Design review of the part built by this model. Coordinates are the model's own, in mm. Round coordinates to 2 decimals unless told otherwise and drop trailing zeros. Order: outer loops, then holes, each group sorted by start corner. A loop starts at its lowest first (then second) coordinate and runs counter-clockwise, first axis right, second up. Notation, with made-up numbers: (-24.5, 34.5) - (26.5, 34.5) arc R14 cw to (26.5, 55.5) - close; hole circle Ø5 at (41, 45.25). An arc over 180 degrees is marked (long way). Write item = value, one per line.
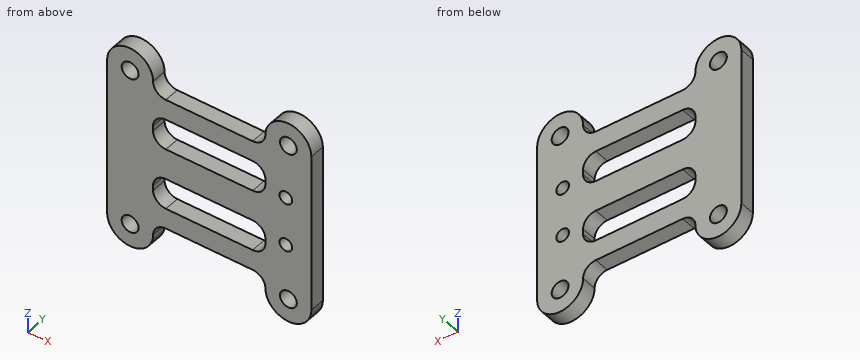
from build123d import *

# Parameters (mm, degrees)
F0_R     = 1.65
F0_R_2   = 1.25
F1_DEPTH = 3


with BuildPart() as f1:
    # F0 (on Front) → F1 (new body)
    with BuildSketch(Plane.XZ):
        with BuildLine():
            ThreePointArc((-8.5, 13), (-10.267767, 13.732233), (-11, 15.5))
            ThreePointArc((-11, 15.5), (-15.5, 20), (-20, 15.5))
            Line((-20, 15.5), (-20, -15.5))
            ThreePointArc((-20, -15.5), (-15.5, -20), (-11, -15.5))
            ThreePointArc((-11, -15.5), (-10.267767, -13.732233), (-8.5, -13))
            Line((-8.5, -13), (8.5, -13))
            ThreePointArc((8.5, -13), (10.267767, -13.732233), (11, -15.5))
            ThreePointArc((11, -15.5), (15.5, -20), (20, -15.5))
            Line((20, -15.5), (20, 15.5))
            ThreePointArc((20, 15.5), (15.5, 20), (11, 15.5))
            ThreePointArc((11, 15.5), (10.267767, 13.732233), (8.5, 13))
            Line((8.5, 13), (-8.5, 13))
        make_face()
        with Locations((-15.5, -15.5)):
            Circle(F0_R, mode=Mode.SUBTRACT)
        with Locations((15.5, -15.5)):
            Circle(F0_R, mode=Mode.SUBTRACT)
        with BuildLine():
            Line((-8.5, -3), (8.5, -3))
            ThreePointArc((8.5, -3), (10.267767, -3.732233), (11, -5.5))
            Line((11, -5.5), (11, -6.5))
            ThreePointArc((11, -6.5), (10.267767, -8.267767), (8.5, -9))
            Line((8.5, -9), (-8.5, -9))
            ThreePointArc((-8.5, -9), (-10.267767, -8.267767), (-11, -6.5))
            Line((-11, -6.5), (-11, -5.5))
            ThreePointArc((-11, -5.5), (-10.267767, -3.732233), (-8.5, -3))
        make_face(mode=Mode.SUBTRACT)
        with Locations((15, -4.75)):
            Circle(F0_R_2, mode=Mode.SUBTRACT)
        with Locations((-15.5, 15.5)):
            Circle(F0_R, mode=Mode.SUBTRACT)
        with BuildLine():
            ThreePointArc((11, 5.5), (10.267767, 3.732233), (8.5, 3))
            Line((8.5, 3), (-8.5, 3))
            ThreePointArc((-8.5, 3), (-10.267767, 3.732233), (-11, 5.5))
            Line((-11, 5.5), (-11, 6.5))
            ThreePointArc((-11, 6.5), (-10.267767, 8.267767), (-8.5, 9))
            Line((-8.5, 9), (8.5, 9))
            ThreePointArc((8.5, 9), (10.267767, 8.267767), (11, 6.5))
            Line((11, 6.5), (11, 5.5))
        make_face(mode=Mode.SUBTRACT)
        with Locations((15, 4.75)):
            Circle(F0_R_2, mode=Mode.SUBTRACT)
        with Locations((15.5, 15.5)):
            Circle(F0_R, mode=Mode.SUBTRACT)
    extrude(amount=F1_DEPTH)


solid = f1.part
Item 1: Take a section at A-A, the plane x = -6.5. State the section outline as (y, z) points.
Data:
outline = (-3, -13) - (0, -13) - (0, -9) - (-3, -9) - close; (-3, -3) - (0, -3) - (0, 3) - (-3, 3) - close; (-3, 9) - (0, 9) - (0, 13) - (-3, 13) - close
Item 2: For line 1 along Z through (x, y) = (5, -0.6); line 2 along Z through (x, y) = (-15.5, -2.35); line 3 along X through (y, z) = (-1.85, -5), list the stretches that pass through material, from the lowest coordinate up. Write a range as [from, to].
Data:
line_1 = [-13, -9], [-3, 3], [9, 13]
line_2 = [-20, -17.15], [-13.85, 13.85], [17.15, 20]
line_3 = [-20, -10.95], [10.95, 13.78], [16.22, 20]
Item 3: Take a section at B-B, the plane z = 8.5. State the section outline as (x, y) points, and give its area (3 significant figures).
Data:
outline = (-20, -3) - (-10, -3) - (-10, 0) - (-20, 0) - close; (10, -3) - (20, -3) - (20, 0) - (10, 0) - close
area = 60.0 mm2
Item 4: Take a section at C-C, the plane y = -1.4. Count the separate pieces of the cut face and the enclosed holes in it, and give its area (3 significant figures).
Data:
separate_pieces = 1
enclosed_holes = 8
area = 965 mm2
Item 5: Insertion check: P1, Ø1, axis at x = -9.5, y = -1.5, coming from the -Z side; P2, Ø1.5, axis at x = 2, y = -1.5, coming from the +Z side; P3, Ø0.9, axis at x = 3, y = -2, coming from the -Z side. Each pin has a flat end and moves straight along its axis. Give the tip position at first contact, or say it passes through.
Data:
P1 = -13.5
P2 = 13
P3 = -13
Item 6: Take a section at D-D, the plane z = -4.75. State the section outline as (x, y) points, and give its area (3 significant figures).
Data:
outline = (-20, -3) - (-10.88, -3) - (-10.88, 0) - (-20, 0) - close; (10.88, -3) - (13.75, -3) - (13.75, 0) - (10.88, 0) - close; (16.25, -3) - (20, -3) - (20, 0) - (16.25, 0) - close
area = 47.2 mm2
